```python
from build123d import *

# Parameters (mm, degrees)
RESSALTO_EXTRUS_O1_DEPTH  = 10
RESSALTO_EXTRUS_O2_DEPTH  = 25
RESSALTO_EXTRUS_O2_TAPER  = 5
RESSALTO_EXTRUS_O3_DEPTH  = 25
RESSALTO_EXTRUS_O3_TAPER  = 10
RESSALTO_EXTRUS_O4_DEPTH  = 25
RESSALTO_EXTRUS_O4_TAPER  = 20
ESBO_O8_R                 = 5
RESSALTO_EXTRUS_O6_DEPTH  = 18
CORTE_EXTRUS_O2_DEPTH     = 2
RESSALTO_EXTRUS_O10_DEPTH = 50
CORTE_EXTRUS_O5_START     = 35
CORTE_EXTRUS_O5_DEPTH     = 50
CORTE_EXTRUS_O6_DEPTH     = 20
CORTE_EXTRUS_O7_DEPTH     = 1
ESBO_O17_R                = 10
CORTE_EXTRUS_O8_DEPTH     = 10


with BuildPart() as part:
    # Esboço1 → Ressalto-extrusão1 (new body)
    with BuildSketch(Plane.XY):
        Polygon((11.714282715, 142.58825066), (-25.240942572, 180.026335933), (-77.844956945, 180.367769505), (-115.283042218, 143.412544218), (-115.624475789, 90.808529845), (-78.669250503, 53.370444572), (-26.06523613, 53.029011), (11.372849143, 89.984236287), align=None)
    extrude(amount=RESSALTO_EXTRUS_O1_DEPTH)

    # Esboço3 → Ressalto-extrusão2 (add)
    with BuildSketch(Plane.XY.offset(10)):
        Polygon((11.372849143, 89.984236287), (11.714282715, 142.58825066), (-25.240942572, 180.026335933), (-77.844956945, 180.367769505), (-115.283042218, 143.412544218), (-115.624475789, 90.808529845), (-78.669250503, 53.370444572), (-26.06523613, 53.029011), align=None)
    extrude(amount=RESSALTO_EXTRUS_O2_DEPTH, taper=RESSALTO_EXTRUS_O2_TAPER)

    # Esboço4 → Ressalto-extrusão3 (add)
    with BuildSketch(Plane.XY.offset(35)):
        Polygon((-26.956995692, 55.222061748), (9.191558856, 90.904388109), (9.521231967, 141.696491098), (-26.161094394, 177.845045645), (-76.953197383, 178.174718757), (-113.10175193, 142.492392396), (-113.431425042, 91.700289407), (-77.749098681, 55.55173486), align=None)
    extrude(amount=RESSALTO_EXTRUS_O3_DEPTH, taper=RESSALTO_EXTRUS_O3_TAPER)

    # Esboço5 → Ressalto-extrusão4 (add)
    with BuildSketch(Plane.XY.offset(60)):
        Polygon((-75.894600212, 59.947965354), (-28.754271643, 59.641994585), (4.795328361, 92.758886578), (5.10129913, 139.899215147), (-28.015592863, 173.448815151), (-75.155921432, 173.75478592), (-108.705521436, 140.637893927), (-109.011492205, 93.497565358), align=None)
    extrude(amount=RESSALTO_EXTRUS_O4_DEPTH, taper=RESSALTO_EXTRUS_O4_TAPER)

    # Esboço8 → Ressalto-extrusão6 (add)
    with BuildSketch(Plane.XY.offset(85)):
        with Locations((-51.955096537, 116.698390253)):
            Circle(ESBO_O8_R)
    extrude(amount=RESSALTO_EXTRUS_O6_DEPTH)

    # Esboço6 → Loft1 section 0
    with BuildSketch(Plane.XY.offset(85)):
        with BuildLine():
            Line((-99.887965086, 97.207462428), (-72.066585693, 69.022566624))
            Line((-72.066585693, 69.022566624), (-32.464168713, 68.765521704))
            Line((-32.464168713, 68.765521704), (-4.279272909, 96.586901097))
            Line((-4.279272909, 96.586901097), (-4.022227989, 136.189318077))
            Line((-4.022227989, 136.189318077), (-31.843607381, 164.374213881))
            Line((-31.843607381, 164.374213881), (-71.446024362, 164.631258801))
            Line((-71.446024362, 164.631258801), (-99.630920166, 136.809879409))
            Line((-99.630920166, 136.809879409), (-99.887965086, 97.207462428))
        make_face()
    # Esboço7 for Loft1 → Loft1 section 1
    with BuildSketch(Plane.XY.offset(103)):
        with BuildLine():
            # circular arc as an exact rational Bezier (weights 1, cos(half-angle), 1)
            Bezier((-72.797833823, 108.223114301), (-69.28725958, 99.58976984), (-60.700212313, 95.967424282), weights=[1, 0.923879532, 1])
            Bezier((-60.700212313, 95.967424282), (-52.113165047, 92.345078724), (-43.479820586, 95.855652967), weights=[1, 0.923879533, 1])
            Bezier((-43.479820586, 95.855652967), (-34.846476125, 99.36622721), (-31.224130567, 107.953274477), weights=[1, 0.923879532, 1])
            Bezier((-31.224130567, 107.953274477), (-27.601785009, 116.540321743), (-31.112359252, 125.173666204), weights=[1, 0.923879533, 1])
            Bezier((-31.112359252, 125.173666204), (-34.622933495, 133.807010665), (-43.209980762, 137.429356223), weights=[1, 0.923879532, 1])
            Bezier((-43.209980762, 137.429356223), (-51.797028028, 141.051701781), (-60.430372489, 137.541127538), weights=[1, 0.923879533, 1])
            Bezier((-60.430372489, 137.541127538), (-69.06371695, 134.030553295), (-72.686062508, 125.443506028), weights=[1, 0.923879532, 1])
            Bezier((-72.686062508, 125.443506028), (-76.308408066, 116.856458762), (-72.797833823, 108.223114301), weights=[1, 0.923879533, 1])
        make_face()
    loft()

    # Esboço9 → Corte-extrusão2 (cut)
    with BuildSketch(Plane.XY.offset(103)):
        with BuildLine():
            ThreePointArc((-44.042402012, 135.456037969), (-51.822961029, 137.056254156), (-59.62363648, 135.557170109))
            ThreePointArc((-59.62363648, 135.557170109), (-66.25684624, 131.187007783), (-70.712744254, 124.611084778))
            ThreePointArc((-70.712744254, 124.611084778), (-72.312960441, 116.830525761), (-70.813876394, 109.02985031))
            ThreePointArc((-70.813876394, 109.02985031), (-66.443714068, 102.39664055), (-59.867791063, 97.940742536))
            ThreePointArc((-59.867791063, 97.940742536), (-52.087232046, 96.340526349), (-44.286556595, 97.839610396))
            ThreePointArc((-44.286556595, 97.839610396), (-37.653346835, 102.209772722), (-33.197448821, 108.785695727))
            ThreePointArc((-33.197448821, 108.785695727), (-31.597232634, 116.566254744), (-33.096316681, 124.366930195))
            ThreePointArc((-33.096316681, 124.366930195), (-37.466479007, 131.000139955), (-44.042402012, 135.456037969))
        make_face()
    extrude(amount=-CORTE_EXTRUS_O2_DEPTH, mode=Mode.SUBTRACT)

    # Esboço13 → Corte-extrusão5 (cut)
    with BuildSketch(Plane.XY.offset(CORTE_EXTRUS_O5_START)):
        Polygon((-98.070713952, 55.683635091), (-5.651465, 55.083775278), (-7.425428207, 63.095457942), (-96.192902738, 63.671615412), align=None)
    extrude(amount=CORTE_EXTRUS_O5_DEPTH, mode=Mode.SUBTRACT)

    # Esboço15 → Corte-extrusão6 (cut)
    with BuildSketch(Plane(origin=(0.409199665, 63.044606215, 0), x_dir=(0.9999789364800716, -0.006490500457210974, 0), z_dir=(-0.006490500457210974, -0.9999789364800716, 0))):
        Polygon((-79.311433136, 61.3), (-60.111433136, 61.3), (-60.111433136, 63.8), (-25.511433136, 63.8), (-25.511433136, 46), (-79.311433136, 46), align=None)
    extrude(amount=-CORTE_EXTRUS_O6_DEPTH, mode=Mode.SUBTRACT)


with BuildPart() as body_2:
    # Esboço12 → Ressalto-extrusão10 (new body)
    with BuildSketch(Plane(origin=(1.167373089, 179.854929138, 0), x_dir=(0.9999789364800716, -0.0064905004572113805, 0), z_dir=(0.0064905004572113805, 0.9999789364800716, 0))):
        Polygon((-79.013994346, 0), (-82.013994346, 0), (-82.013994346, -61.615746699), (-64.879741046, -78.75), (-40.648247647, -78.75), (-23.513994346, -61.615746699), (-23.513994346, 0), (-26.408871925, 0), (-26.408871925, -10), (-26.513994346, -10), (-26.513994346, -60.373106012), (-41.890888334, -75.75), (-63.637100359, -75.75), (-79.013994346, -60.373106012), (-79.013994346, -10), align=None)
    extrude(amount=-RESSALTO_EXTRUS_O10_DEPTH)


with BuildPart() as corte_extrus_o7_tool:
    # Esboço16 → Corte-extrusão7 (new body)
    with BuildSketch(Plane(origin=(1.167373089, 179.854929138, 0), x_dir=(0.9999789364800716, -0.0064905004572113805, 0), z_dir=(0.0064905004572113805, 0.9999789364800716, 0))):
        Polygon((-26.408871925, 0), (-79.013994346, 0), (-79.013994346, -10), (-78.108019572, -35), (-27.314846699, -35), (-26.408871925, -10), align=None)
    extrude(amount=-CORTE_EXTRUS_O7_DEPTH)


with BuildPart() as part_1:
    add(part.part)

    # Corte-extrusão7: cut by corte_extrus_o7_tool
    add(corte_extrus_o7_tool.part, mode=Mode.SUBTRACT)

    # Esboço17 → Corte-extrusão8 (cut)
    with BuildSketch(Plane(origin=(1.160882588, 178.854950202, 0), x_dir=(0.9999789364800716, -0.0064905004572113805, 0), z_dir=(0.0064905004572113805, 0.9999789364800716, 0))):
        with Locations(Location((-39.763994346, -27.25, 0), (0, 0, 180))):
            Circle(ESBO_O17_R)
        with Locations(Location((-65.763994346, -27.25, 0), (0, 0, 180))):
            Circle(ESBO_O17_R)
    extrude(amount=-CORTE_EXTRUS_O8_DEPTH, mode=Mode.SUBTRACT)


with BuildPart() as body_2_1:
    add(body_2.part)

    # Corte-extrusão7: cut by corte_extrus_o7_tool
    add(corte_extrus_o7_tool.part, mode=Mode.SUBTRACT)


with BuildPart() as part_2:
    add(part_1.part)

    # Combinar1: union body 2
    add(body_2_1.part)


solid = part_2.part
```
Work out the finished part from the listing and answer in its coordinate system (mm). A direction names the side the tool comes from. Coordinates: 2 decimals unless noted, no trailing zeros. Loops run counter-clockwise (first coordinate to the right, second up) from the corner with the lowest first, then second, coordinate; pieces in that order, holes last.
1) For a pull along Z with two mould halves and no side action, classify faces 1 (the flat face through (-76.685, 174.697, 50.103)), 2 (the flat face through (-52, 174, 78.75)) as +Z half, -Z half, draft (parallel to the pull), parting line (faces both ways), or undercut.
Results:
face 1: undercut
face 2: +Z half
2) For faces 3 (the flat face through (-52, 73, 46)), 4 (the flat face through (-52, 117, 101)), determine the directions among +Z, -Z, +X, -X, +Y, -Y from which every point of the face is accessible in a straight line to the end or side of a thin tool.
Results:
face 3: -Y
face 4: +Z
3) Flat-ended cylindrical pins translate along their axes: pin 1 (6 mm diameter, centred on x = -92, z = 84.5, fed in from -Y); pin 2 (2.5 mm diameter, centred on x = -67, y = 60, fed in from +Z); pin 3 (1.5 mm diameter, centred on x = -50, y = 163.5, fed in from +Z). Find the tip coordinate at first contact, or state that the pin passes through.
Results:
pin 1: stops at y = 85.54
pin 2: stops at z = 35
pin 3: stops at z = 86.24
4) Section B-B (x = 1) is taken. Give the vertices of the cut face in (y, z), plus the area to 3 significant figures.
Results:
outline: (79.75, 0) - (153.44, 0) - (153.44, 10) - (150.33, 35) - (144.05, 60) - (138.23, 71.24) - (94.36, 70.46) - (89.01, 60) - (82.82, 35) - (79.75, 10) - close
area: 4,570 mm2
5) Section D-D (z = 83) is taken. Give the vertices of the cut face in (x, y), plus the area to 3 significant figures.
Results:
outline: (-100.62, 96.91) - (-72.37, 68.3) - (-32.17, 68.04) - (-3.55, 96.28) - (-3.29, 136.49) - (-31.54, 165.1) - (-71.74, 165.36) - (-100.36, 137.12) - close
area: 7,810 mm2
6) Consider probe 1 along Z at (x, y) = (-90, 157.5); probe 2 along Z at (x, y) = (-49, 80.5); probe 3 along Y at (x, z) = (4, 20). Determine where each line is inside the solid, lowest interval first.
Results:
probe 1: z = 0 to 63.13
probe 2: z = 0 to 46, 63.8 to 93.24
probe 3: y = 83.94 to 149.16
7) Section A-A (z = 30) is taken. Give the vertices of the cut face in (x, y), plus the area to 3 significant figures.
Results:
outline: (-113.87, 91.52) - (-77.93, 55.12) - (-26.78, 54.78) - (9.63, 90.72) - (9.96, 141.87) - (-22.38, 174.64) - (-22.35, 180.01) - (-25.35, 180.03) - (-25.36, 177.66) - (-25.98, 178.28) - (-28.99, 178.3) - (-29.05, 169.05) - (-48.28, 169.18) - (-48.22, 178.43) - (-54.99, 178.47) - (-55.05, 169.22) - (-74.28, 169.34) - (-74.22, 178.59) - (-77.13, 178.61) - (-77.86, 177.89) - (-77.84, 180.37) - (-80.84, 180.39) - (-80.88, 174.91) - (-113.54, 142.68) - close
area: 12,300 mm2
8) Section C-C (z = 58) is taken. Give the vertices of the cut face in (x, y), plus the area to 3 significant figures.
Results:
outline: (-109.37, 93.35) - (-79.96, 63.57) - (-78.9, 63.56) - (-78.77, 83.56) - (-24.97, 83.21) - (-25.1, 63.21) - (-24.64, 63.21) - (5.15, 92.61) - (5.45, 140.04) - (-22.42, 168.28) - (-22.35, 180.01) - (-25.35, 180.03) - (-25.4, 171.3) - (-27.87, 173.8) - (-75.3, 174.11) - (-77.9, 171.54) - (-77.84, 180.37) - (-80.84, 180.39) - (-80.92, 168.56) - (-109.06, 140.79) - close
area: 9,650 mm2
